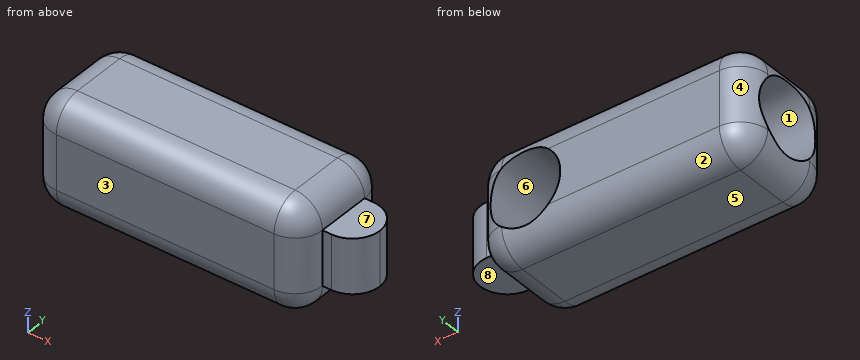
```python
from build123d import *

# Parameters (mm, degrees)
SKETCH1_W           = 150
SKETCH1_H           = 60
BOSS_EXTRUDE3_DEPTH = 60
SKETCH3_R           = 20
CUT_EXTRUDE1_DEPTH  = 100
FILLET1_R           = 15
SKETCH5_R           = 20
CUT_EXTRUDE2_DEPTH  = 40
SKETCH6_W           = 30
SKETCH6_H           = 30
BOSS_EXTRUDE4_DEPTH = 20
FILLET4_R           = 15
FILLET5_R           = 15


# Some blends are built 0.0001 mm under size
with BuildPart() as part:
    # Sketch1 → Boss-Extrude3 (new body)
    with BuildSketch(Plane(origin=(0, 0, 0), x_dir=(1, 0, 0), z_dir=(0, 1, 0))):
        Rectangle(SKETCH1_W, SKETCH1_H)
    extrude(amount=BOSS_EXTRUDE3_DEPTH)

    # Sketch3 → Cut-Extrude1 (cut)
    with BuildSketch(Plane.ZY.offset(75)):
        with Locations((0, 30)):
            Circle(SKETCH3_R)
    extrude(amount=-CUT_EXTRUDE1_DEPTH, mode=Mode.SUBTRACT)

    # Fillet1
    # the kernel refuses this fillet: 15 mm, written as the material it takes off along each edge
    with BuildSketch(Plane(origin=(-60, 45, 15), x_dir=(0, 1, 0), z_dir=(-1, 0, 0))) as fillet1_piece_1_section:
        Polygon((0, 0), (FILLET1_R, 0), (FILLET1_R, -FILLET1_R), (0, -FILLET1_R), align=None)
    fillet1_piece_1 = extrude(amount=FILLET1_R, mode=Mode.PRIVATE)
    fillet1_piece_1 = fillet1_piece_1 - Plane(origin=(-60, 45, 15), x_dir=(0, -0.7071067811865475, -0.7071067811865475), z_dir=(-1, 0, 0)) * Sphere(FILLET1_R, mode=Mode.PRIVATE)
    add(fillet1_piece_1, mode=Mode.SUBTRACT)
    with BuildSketch(Plane(origin=(-60, 45, -15), x_dir=(-1, 0, 0), z_dir=(0, 0, -1))) as fillet1_piece_2_section:
        Polygon((0, 0), (FILLET1_R, 0), (FILLET1_R, FILLET1_R), (0, FILLET1_R), align=None)
    fillet1_piece_2 = extrude(amount=FILLET1_R, mode=Mode.PRIVATE)
    fillet1_piece_2 = fillet1_piece_2 - Plane(origin=(-60, 45, -15), x_dir=(0.7071067811865475, -0.7071067811865475, 0), z_dir=(0, 0, -1)) * Sphere(FILLET1_R, mode=Mode.PRIVATE)
    add(fillet1_piece_2, mode=Mode.SUBTRACT)
    with BuildSketch(Plane(origin=(60, 45, 15), x_dir=(0, 1, 0), z_dir=(1, 0, 0))) as fillet1_piece_3_section:
        Polygon((0, 0), (FILLET1_R, 0), (FILLET1_R, FILLET1_R), (0, FILLET1_R), align=None)
    fillet1_piece_3 = extrude(amount=FILLET1_R, mode=Mode.PRIVATE)
    fillet1_piece_3 = fillet1_piece_3 - Plane(origin=(60, 45, 15), x_dir=(0, -0.7071067811865475, -0.7071067811865475), z_dir=(1, 0, 0)) * Sphere(FILLET1_R, mode=Mode.PRIVATE)
    add(fillet1_piece_3, mode=Mode.SUBTRACT)
    with BuildSketch(Plane(origin=(60, 45, -15), x_dir=(1, 0, 0), z_dir=(0, 0, -1))) as fillet1_piece_4_section:
        Polygon((0, 0), (FILLET1_R, 0), (FILLET1_R, -FILLET1_R), (0, -FILLET1_R), align=None)
    fillet1_piece_4 = extrude(amount=FILLET1_R, mode=Mode.PRIVATE)
    fillet1_piece_4 = fillet1_piece_4 - Plane(origin=(60, 45, -15), x_dir=(-0.7071067811865475, -0.7071067811865475, 0), z_dir=(0, 0, -1)) * Sphere(FILLET1_R, mode=Mode.PRIVATE)
    add(fillet1_piece_4, mode=Mode.SUBTRACT)
    with BuildSketch(Plane(origin=(60, 15, 15), x_dir=(0, -1, 0), z_dir=(1, 0, 0))) as fillet1_piece_5_section:
        Polygon((0, 0), (FILLET1_R, 0), (FILLET1_R, -FILLET1_R), (0, -FILLET1_R), align=None)
    fillet1_piece_5 = extrude(amount=FILLET1_R, mode=Mode.PRIVATE)
    fillet1_piece_5 = fillet1_piece_5 - Plane(origin=(60, 15, 15), x_dir=(0, 0.7071067811865475, -0.7071067811865475), z_dir=(1, 0, 0)) * Sphere(FILLET1_R, mode=Mode.PRIVATE)
    add(fillet1_piece_5, mode=Mode.SUBTRACT)
    with BuildSketch(Plane(origin=(-60, 15, 15), x_dir=(0, -1, 0), z_dir=(-1, 0, 0))) as fillet1_piece_6_section:
        Polygon((0, 0), (FILLET1_R, 0), (FILLET1_R, FILLET1_R), (0, FILLET1_R), align=None)
    fillet1_piece_6 = extrude(amount=FILLET1_R, mode=Mode.PRIVATE)
    fillet1_piece_6 = fillet1_piece_6 - Plane(origin=(-60, 15, 15), x_dir=(0, 0.7071067811865475, -0.7071067811865475), z_dir=(-1, 0, 0)) * Sphere(FILLET1_R, mode=Mode.PRIVATE)
    add(fillet1_piece_6, mode=Mode.SUBTRACT)
    with BuildSketch(Plane(origin=(-60, 15, -15), x_dir=(-1, 0, 0), z_dir=(0, 0, -1))) as fillet1_piece_7_section:
        Polygon((0, 0), (FILLET1_R, 0), (FILLET1_R, -FILLET1_R), (0, -FILLET1_R), align=None)
    fillet1_piece_7 = extrude(amount=FILLET1_R, mode=Mode.PRIVATE)
    fillet1_piece_7 = fillet1_piece_7 - Plane(origin=(-60, 15, -15), x_dir=(0.7071067811865475, 0.7071067811865475, 0), z_dir=(0, 0, -1)) * Sphere(FILLET1_R, mode=Mode.PRIVATE)
    add(fillet1_piece_7, mode=Mode.SUBTRACT)
    with BuildSketch(Plane(origin=(60, 15, -15), x_dir=(1, 0, 0), z_dir=(0, 0, -1))) as fillet1_piece_8_section:
        Polygon((0, 0), (FILLET1_R, 0), (FILLET1_R, FILLET1_R), (0, FILLET1_R), align=None)
    fillet1_piece_8 = extrude(amount=FILLET1_R, mode=Mode.PRIVATE)
    fillet1_piece_8 = fillet1_piece_8 - Plane(origin=(60, 15, -15), x_dir=(-0.7071067811865475, 0.7071067811865475, 0), z_dir=(0, 0, -1)) * Sphere(FILLET1_R, mode=Mode.PRIVATE)
    add(fillet1_piece_8, mode=Mode.SUBTRACT)
    with BuildSketch(Plane(origin=(-75, 60, 15), x_dir=(0, -1, 0), z_dir=(0, 0, -1)), Plane(origin=(75, 60, -15), x_dir=(0, -1, 0), z_dir=(0, 0, 1)), Plane(origin=(-75, 15, 30), x_dir=(0, 0, -1), z_dir=(0, 1, 0)), Plane(origin=(-75, 15, -30), x_dir=(1, 0, 0), z_dir=(0, 1, 0))) as fillet1_piece_9:
        with BuildLine():
            CenterArc((FILLET1_R, -FILLET1_R), FILLET1_R, 90, 90)
            Line((0, -FILLET1_R), (0, 0))
            Line((0, 0), (FILLET1_R, 0))
        make_face()
    extrude(amount=30, mode=Mode.SUBTRACT)
    with BuildSketch(Plane(origin=(60, 60, 30), x_dir=(0, 0, -1), z_dir=(-1, 0, 0)), Plane(origin=(-60, 0, -30), x_dir=(0, 1, 0), z_dir=(1, 0, 0))) as fillet1_piece_10:
        with BuildLine():
            CenterArc((FILLET1_R, FILLET1_R), FILLET1_R, 180, 90)
            Line((0, FILLET1_R), (0, 0))
            Line((0, 0), (FILLET1_R, 0))
        make_face()
    extrude(amount=120, mode=Mode.SUBTRACT)
    with BuildSketch(Plane(origin=(60, 0, 30), x_dir=(0, 0, -1), z_dir=(-1, 0, 0)), Plane(origin=(-60, 60, -30), x_dir=(0, -1, 0), z_dir=(1, 0, 0))) as fillet1_piece_11:
        with BuildLine():
            CenterArc((FILLET1_R, -FILLET1_R), FILLET1_R, 90, 90)
            Line((0, -FILLET1_R), (0, 0))
            Line((0, 0), (FILLET1_R, 0))
        make_face()
    extrude(amount=120, mode=Mode.SUBTRACT)
    with BuildSketch(Plane(origin=(-75, 0, 15), x_dir=(0, 1, 0), z_dir=(0, 0, -1)), Plane(origin=(75, 0, -15), x_dir=(0, 1, 0), z_dir=(0, 0, 1)), Plane(origin=(75, 15, 30), x_dir=(0, 0, -1), z_dir=(0, 1, 0)), Plane(origin=(75, 15, -30), x_dir=(-1, 0, 0), z_dir=(0, 1, 0))) as fillet1_piece_12:
        with BuildLine():
            CenterArc((FILLET1_R, FILLET1_R), FILLET1_R, 180, 90)
            Line((0, FILLET1_R), (0, 0))
            Line((0, 0), (FILLET1_R, 0))
        make_face()
    extrude(amount=30, mode=Mode.SUBTRACT)

    # Sketch5 → Cut-Extrude2 (cut)
    with BuildSketch(Plane(origin=(0, 60, 0), x_dir=(1, 0, 0), z_dir=(0, 1, 0))):
        with Locations(Location((47.646230656, 0, 0), (0, 0, 270))):
            Circle(SKETCH5_R)
    extrude(amount=-CUT_EXTRUDE2_DEPTH, mode=Mode.SUBTRACT)

    # Sketch6 → Boss-Extrude4 (add)
    with BuildSketch(Plane(origin=(75, 0, 0), x_dir=(0, 0, -1), z_dir=(1, 0, 0))):
        with Locations((0, 30)):
            Rectangle(SKETCH6_W, SKETCH6_H)
    extrude(amount=BOSS_EXTRUDE4_DEPTH)

    # Fillet4
    fillet4_edges = [part.edges().sort_by_distance(p)[0] for p in [
        (95, 15, 0),
    ]]
    fillet(fillet4_edges, radius=FILLET4_R)

    # Fillet5
    fillet5_edges = [part.edges().sort_by_distance(p)[0] for p in [
        (95, 45, 0),
    ]]
    fillet(fillet5_edges, radius=FILLET5_R - 0.0001)  # a hair under: the kernel refuses the full size


solid = part.part
```
The model under review builds one solid part; all positions refer to its coordinate system, in mm. Face numbers are marked on the shaded views. A direction names the side the tool comes from. Round coordinates to 2 decimals unless told otherwise and drop trailing zeros. Order: outer loops, then holes, each group sorted by start corner. A loop starts at its lowest first (then second) coordinate and runs counter-clockwise, first axis right, second up. Notation, with made-up numbers: M 24.25,43 L 80.25,43 A13 ccw 80.25,49 Z; hole C 53,57.25 d4. An arc over 180 degrees is marked long. Use a Markdown table: item, result.
1) Insertion check: pin 1 (6 mm diameter, centred on x = 66, y = 7.5, fed in from -Z); pin 2 (20 mm diameter, centred on y = 33.5, z = 5, fed in from -X); pin 3 (6 mm diameter, centred on x = 29, y = 6.5, fed in from +Z). Each pin has a flat end and moves straight along its axis. Give the tip position at first contact, or say it passes through.
Report:
| item | result |
|---|---|
| pin 1 | z = -28.47 |
| pin 2 | x = 25 |
| pin 3 | z = 28.96 |
2) Consider section C-C (x = 44.5). Write out the cut boundary in (y, z).
Report:
| item | result |
|---|---|
| outline | M 0,-15 A15 ccw 15,-30 L 45,-30 A15 ccw 59.23,-19.75 L 20,-19.75 L 20,19.75 L 59.23,19.75 A15 ccw 45,30 L 15,30 A15 ccw 0,15 Z |
3) Wall thickness on line 1 along Y through (x, z) = (77, 13); line 2 along X through (y, z) = (20.5, -10.5); line 3 along Y through (x, z) = (-13, 4): over which ranges is each line inside the solid? List them lowest first. Write a range as [from, to].
Report:
| item | result |
|---|---|
| line 1 | [15, 45] |
| line 2 | [25, 30.62], [64.67, 91.61] |
| line 3 | [0, 10.4], [49.6, 60] |
4) Consider section B-B (y = 33). Write out the cut boundary in (x, z), then the cut area to 3 significant figures.
Report:
| item | result |
|---|---|
| outline | M -74.22,-19.77 A15 ccw -60,-30 L 60,-30 A15 ccw 75,-15 L 94.7,-15 L 94.7,15 L 75,15 A15 ccw 60,30 L -60,30 A15 ccw -74.22,19.77 L 25,19.77 L 25,-19.77 Z; hole C 47.65,0 d40 |
| area | 4,190 mm^2 |
5) Draft analysis for pull direction Y (two halves, no side actions). For the marked faces 1, 2 and 3, state which applies: released by +Y, released by -Y, zero draft, split by the parting line, or undercut.
Report:
| item | result |
|---|---|
| face 1 | undercut |
| face 2 | released by +Y |
| face 3 | released by -Y |
6) Consider section A-A (x = 16). Write out the cut boundary in (y, z).
Report:
| item | result |
|---|---|
| outline | M 0,-15 A15 ccw 15,-30 L 45,-30 A15 ccw 60,-15 L 60,15 A15 ccw 45,30 L 15,30 A15 ccw 0,15 Z; hole C 30,0 d40 |
7) Tool access review of the marked faces 4, 5, 6, 7 and 8: name each direction out of +Z, -Z, +X, -X, +Y, -Y from which nothing blocks a thin tool from reaching the whole face with its end or side.
Report:
| item | result |
|---|---|
| face 4 | +Z, -Z, -X, +Y |
| face 5 | -Z, +X, -X, +Y, -Y |
| face 6 | +Y |
| face 7 | +Z, +X, +Y, -Y |
| face 8 | -Z, +X, +Y, -Y |
